from build123d import *

# Parameters (mm, degrees)
ESQUISSE1_W             = 55
ESQUISSE1_H             = 40
EXTRUSION1_DEPTH        = 40
ESQUISSE2_W             = 8
ESQUISSE2_H             = 8
ENL_V_MAT_EXTRU_1_DEPTH = 41
ENL_V_MAT_EXTRU_2_DEPTH = 40
ENL_V_MAT_EXTRU_3_DEPTH = 40
ENL_V_MAT_EXTRU_4_DEPTH = 40
ESQUISSE6_R             = 8
ENL_V_MAT_EXTRU_5_DEPTH = 41
ESQUISSE7_R             = 14
ENL_V_MAT_EXTRU_6_DEPTH = 20


with BuildPart() as part:
    # Esquisse1 → Extrusion1 (new body)
    with BuildSketch(Plane.XY):
        with Locations((-21.875589067, 0.118096136)):
            Rectangle(ESQUISSE1_W, ESQUISSE1_H)
    extrude(amount=EXTRUSION1_DEPTH)

    # Esquisse2 → Enlèv. mat.-Extru.1 (cut, through all)
    with BuildSketch(Plane.XY.offset(40)):
        with Locations((1.624410933, -15.881903864)):
            Rectangle(ESQUISSE2_W, ESQUISSE2_H)
    extrude(amount=-ENL_V_MAT_EXTRU_1_DEPTH, mode=Mode.SUBTRACT)

    # Esquisse3 → Enlèv. mat.-Extru.2 (cut)
    with BuildSketch(Plane.XY.offset(40)):
        Polygon((-49.375589067, -3.881903864), (-34.375589067, -3.881903864), (-34.375589067, -11.881903864), (-26.375589067, -11.881903864), (-26.375589067, -19.881903864), (-49.375589067, -19.881903864), align=None)
    extrude(amount=-ENL_V_MAT_EXTRU_2_DEPTH, mode=Mode.SUBTRACT)

    # Esquisse4 → Enlèv. mat.-Extru.3 (cut)
    with BuildSketch(Plane(origin=(0, 20.118096136, 0), x_dir=(-1, 0, 0), z_dir=(0, 1, 0))):
        Polygon((49.375589067, 0), (39.375589067, 0), (49.375589067, 10), align=None)
    extrude(amount=-ENL_V_MAT_EXTRU_3_DEPTH, mode=Mode.SUBTRACT)

    # Esquisse5 → Enlèv. mat.-Extru.4 (cut)
    with BuildSketch(Plane(origin=(0, 20.118096136, 0), x_dir=(-1, 0, 0), z_dir=(0, 1, 0))):
        Polygon((49.375589067, 30), (39.375589067, 40), (49.375589067, 40), align=None)
    extrude(amount=-ENL_V_MAT_EXTRU_4_DEPTH, mode=Mode.SUBTRACT)

    # Esquisse6 → Enlèv. mat.-Extru.5 (cut, through all)
    with BuildSketch(Plane(origin=(0, 20.118096136, 0), x_dir=(-1, 0, 0), z_dir=(0, 1, 0))):
        with Locations((14.375589067, 20)):
            Circle(ESQUISSE6_R)
    extrude(amount=-ENL_V_MAT_EXTRU_5_DEPTH, mode=Mode.SUBTRACT)

    # Esquisse7 → Enlèv. mat.-Extru.6 (cut)
    with BuildSketch(Plane(origin=(0, 20.118096136, 0), x_dir=(-1, 0, 0), z_dir=(0, 1, 0))):
        with Locations((14.375589067, 20)):
            Circle(ESQUISSE7_R)
    extrude(amount=-ENL_V_MAT_EXTRU_6_DEPTH, mode=Mode.SUBTRACT)


solid = part.part
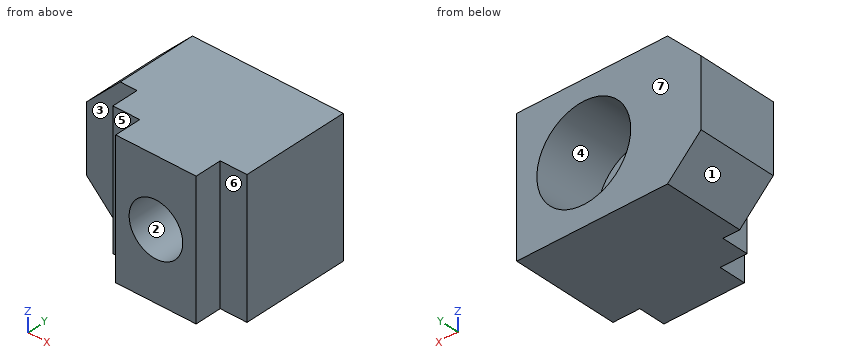
The model under review builds one solid part; all positions refer to its coordinate system, in mm. Face numbers are marked on the shaded views. A direction names the side the tool comes from. Coordinates: 2 decimals unless noted, no trailing zeros. Loops run counter-clockwise (first coordinate to the right, second up) from the corner with the lowest first, then second, coordinate; pieces in that order, holes last.
(1) Consider section A-A, the plane z = 20. Give the boundary of the cut face in (x, y).
Determined:
outline: (-49.38, -3.88) - (-34.38, -3.88) - (-34.38, -11.88) - (-26.38, -11.88) - (-26.38, -19.88) - (-22.38, -19.88) - (-22.38, 0.12) - (-28.38, 0.12) - (-28.38, 20.12) - (-49.38, 20.12) - close; (-6.38, -19.88) - (-2.38, -19.88) - (-2.38, -11.88) - (5.62, -11.88) - (5.62, 20.12) - (-0.38, 20.12) - (-0.38, 0.12) - (-6.38, 0.12) - close
(2) Consider section C-C, the plane z = 4. Give the boundary of the cut face in (x, y).
Determined:
outline: (-43.38, -3.88) - (-34.38, -3.88) - (-34.38, -11.88) - (-26.38, -11.88) - (-26.38, -19.88) - (-2.38, -19.88) - (-2.38, -11.88) - (5.62, -11.88) - (5.62, 20.12) - (-43.38, 20.12) - close
(3) Tool access review of the marked faces 4, 5, 6 and 7: name each direction out of +Z, -Z, +X, -X, +Y, -Y from which nothing blocks a thin tool from reaching the whole face with its end or side.
Determined:
face 4: +Y
face 5: +Z, -Z, -X, -Y
face 6: +Z, -Z, +X, -Y
face 7: +Z, -Z, +X, -X, +Y
(4) Draft analysis for pull direction X (two halves, no side actions). For the marked faces 1, 2 and 3, state which applies: +X half, -X half, draft (parallel to the pull), parting line (faces both ways), or undercut.
Determined:
face 1: -X half
face 2: undercut
face 3: draft
(5) Wall thickness on L1, parallel to Y at x = -35.5, z = 33.5; L2, parallel to X at y = -13, z = 35; L3, parallel to Z at x = -12, y = -3.5: over which ranges is each line inside the solid? List them lowest first.
Determined:
L1: y = -3.88 to 20.12
L2: x = -26.38 to -2.38
L3: z = 0 to 12.36, 27.64 to 40
(6) Consider section D-D, the plane x = -4.5. Give the boundary of the cut face in (y, z), plus the area to 3 significant figures.
Determined:
outline: (-19.88, 0) - (20.12, 0) - (20.12, 10.08) - (0.12, 10.08) - (0.12, 29.92) - (20.12, 29.92) - (20.12, 40) - (-19.88, 40) - close
area: 1,200 mm2
(7) Insertion check: P1, Ø6.5, axis at y = -17.5, z = 20.5, coming from the -X side; P2, Ø2.5, axis at y = -17, z = 23.5, coming from the +X side; P3, Ø1.5, axis at x = -12, z = 27, coming from the +Y side. Each pin has a flat end and moves straight along its axis. Give the tip position at first contact, or say it passes through.
Determined:
P1: stops at x = -26.38
P2: stops at x = -2.38
P3: stops at y = 0.12
(8) Consider section B-B, the plane y = 11. Give the boundary of the cut face in (x, z).
Determined:
outline: (-49.38, 10) - (-39.38, 0) - (5.62, 0) - (5.62, 40) - (-39.38, 40) - (-49.38, 30) - close; hole circle Ø28 at (-14.38, 20)
